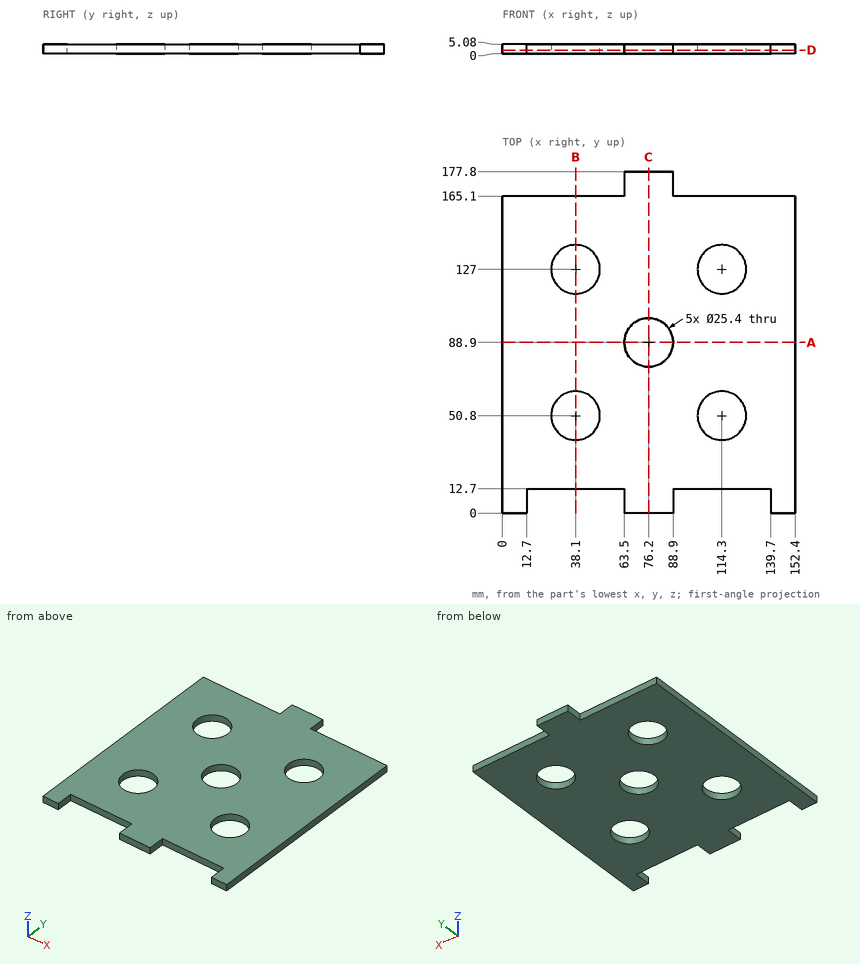
Study the drawing (mm; zero at the part's minimum x, y, z) and answer. Round coordinates to 2 decimals unless told otherwise and drop trailing zeros. Write each loop counter-clockwise with the first axis right and the second up, starting at its lowest first coordinate (ties: lowest second). Pieces come first, ordered by that corner, then holes.
1) Flat-ended cylindrical pins translate along their axes: P1, Ø1.5, axis at x = 45, z = 3.5, coming from the -Y side; P2, Ø1, axis at x = 37, z = 1.5, coming from the +Y side; P3, Ø2.5, axis at y = 6, z = 3, coming from the -X side; P4, Ø2.5, axis at y = 173.5, z = 2.5, coming from the +X side. Find the tip coordinate at first contact, or state that the pin passes through.
2) Consider probe 1 along Y at (x, z) = (114.3, 1.75); probe 2 along X at (y, z) = (130, 2.95); probe 3 along Y at (x, z) = (76.2, 2.2). Determine where each line is inside the solid, lowest interval first.
3) A cutting plane is placed at A-A on y = 88.9. Determine the outline of the cut face in (x, z), and give its area (3 significant figures).
4) A cutting plane is placed at D-D on z = 1.9. Determine the outline of the cut face in (x, y).
5) A cutting plane is placed at C-C on x = 76.2. Determine the outline of the cut face in (y, z).
6) A cutting plane is placed at B-B on x = 38.1. Determine the outline of the cut face in (y, z), and give its area (3 significant figures).
Entries:
1. P1: stops at y = 12.7
1. P2: stops at y = 165.1
1. P3: stops at x = 0
1. P4: stops at x = 88.9
2. probe 1: y = 12.7 to 38.1, 63.5 to 114.3, 139.7 to 165.1
2. probe 2: x = 0 to 25.76, 50.44 to 101.96, 126.64 to 152.4
2. probe 3: y = 0 to 76.2, 101.6 to 177.8
3. outline: (0, 0) - (63.5, 0) - (63.5, 5.08) - (0, 5.08) - close; (88.9, 0) - (152.4, 0) - (152.4, 5.08) - (88.9, 5.08) - close
3. area: 645 mm2
4. outline: (0, 0) - (12.7, 0) - (12.7, 12.7) - (63.5, 12.7) - (63.5, 0) - (88.9, 0) - (88.9, 12.7) - (139.7, 12.7) - (139.7, 0) - (152.4, 0) - (152.4, 165.1) - (88.9, 165.1) - (88.9, 177.8) - (63.5, 177.8) - (63.5, 165.1) - (0, 165.1) - close; hole circle Ø25.4 at (38.1, 50.8); hole circle Ø25.4 at (38.1, 127); hole circle Ø25.4 at (76.2, 88.9); hole circle Ø25.4 at (114.3, 50.8); hole circle Ø25.4 at (114.3, 127)
5. outline: (0, 0) - (76.2, 0) - (76.2, 5.08) - (0, 5.08) - close; (101.6, 0) - (177.8, 0) - (177.8, 5.08) - (101.6, 5.08) - close
6. outline: (12.7, 0) - (38.1, 0) - (38.1, 5.08) - (12.7, 5.08) - close; (63.5, 0) - (114.3, 0) - (114.3, 5.08) - (63.5, 5.08) - close; (139.7, 0) - (165.1, 0) - (165.1, 5.08) - (139.7, 5.08) - close
6. area: 516 mm2
